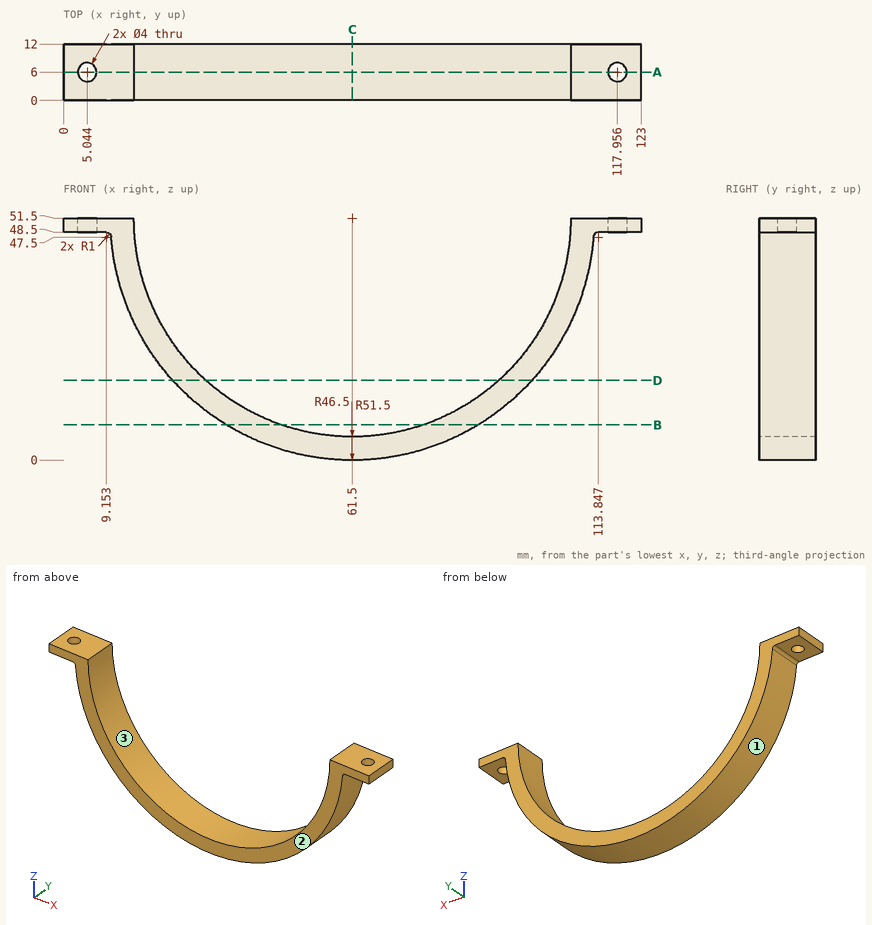
Geometry: see drawing. Coordinates: mm, zero at the bounding-box minimum. Round coordinates to 2 decimals unless told otherwise and drop trailing zeros. Write each loop counter-clockwise with the first axis right and the second up, starting at its lowest first coordinate (ties: lowest second). Pieces come first, ordered by that corner, then holes. Notation, with made-up numbers: M 49.25,49 L 80.25,49 A16 cw 80.25,55 Z; hole C -7.5,21.5 d4. An arc over 180 degrees is marked long. Answer in a Markdown table with one row per item. Add a question column.
(1) Cut plane C-C, the plane x = 61.5. Return the cut outline in (y, z), then the cut area to 3 significant figures.
(2) Draft query along X for the marked faces 1, 2 and 3. Return one class per face: pulls with the +X half, pulls with the -X half, needs draft (parallel to the pull), parting line crosses it, or undercut.
(3) Contact query for flat-ended pins moving along their axis: pin 1 (4 mm diameter, centred on y = 3.5, z = 8.5, fed in from +X) (1 decimal); pin 2 (2.5 mm diameter, centred on x = 2.5, y = 5.5, fed in from -Z); pin 3 (5 mm diameter, centred on x = 104, y = 10.5, fed in from -Z). Output: stop coordinate, or through.
(4) Cut plane A-A, the plane y = 6. Return the cut outline in (x, z).
(5) Ray query, L1, parallel to X at y = 9, z = 14.5 (1 decimal); L2, parallel to X at y = 4.5, z = 32 (1 decimal); L3, parallel to Z at x = 115.5, y = 1.25. Return the intervals inside material, ascending.
(6) Cut plane B-B, the plane z = 7.5. Return the cut outline in (x, y), then the cut area to 3 significant figures.
(7) Cut plane D-D, the plane z = 17. Return the cut outline in (x, y), then the cut area to 3 significant figures.
Established:
| question | item | result |
|---|---|---|
| 1 | outline | M 0,0 L 12,0 L 12,5 L 0,5 Z |
| 1 | area | 60.0 mm² |
| 2 | face 1 | parting line crosses it |
| 2 | face 2 | needs draft |
| 2 | face 3 | undercut |
| 3 | pin 1 | x = 92.7 |
| 3 | pin 2 | z = 48.5 |
| 3 | pin 3 | z = 19.06 |
| 4 | outline | M 0,48.5 L 3.04,48.5 L 3.04,51.5 L 0,51.5 Z; M 7.04,48.5 L 9.15,48.5 A1 cw 10.15,47.58 A51.5 ccw 112.85,47.58 A1 cw 113.85,48.5 L 115.96,48.5 L 115.96,51.5 L 108,51.5 A46.5 cw 15,51.5 L 7.04,51.5 Z; M 119.96,48.5 L 123,48.5 L 123,51.5 L 119.96,51.5 Z |
| 5 | L1 | 25.7 to 33.3, 89.7 to 97.3 |
| 5 | L2 | 13.8 to 19.3, 103.7 to 109.2 |
| 5 | L3 | 48.5 to 51.5 |
| 6 | outline | M 34.74,0 L 46.46,0 L 46.46,12 L 34.74,12 Z; M 76.54,0 L 88.26,0 L 88.26,12 L 76.54,12 Z |
| 6 | area | 281 mm² |
| 7 | outline | M 23.26,0 L 30.32,0 L 30.32,12 L 23.26,12 Z; M 92.68,0 L 99.74,0 L 99.74,12 L 92.68,12 Z |
| 7 | area | 169 mm² |
